Work out the finished part from the listing and answer in its coordinate system (mm). Round coordinates to 2 decimals unless told otherwise and drop trailing zeros. Loops run counter-clockwise (first coordinate to the right, second up) from the corner with the lowest first, then second, coordinate; pieces in that order, holes last. Notation, with made-up numbers: (76.5, -9.5) - (96.5, -9.5) arc R14 ccw to (96.5, 11.5) - close; hole circle Ø7 at (-30, -40). An arc over 180 degrees is marked (long way). Answer as CSV lines item,"result". Start each with the question number.
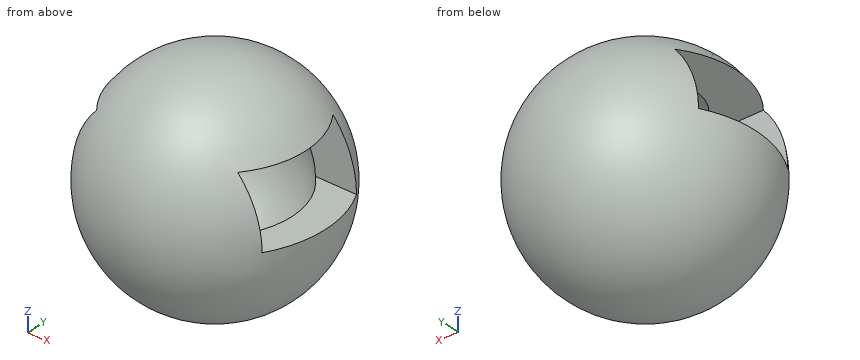
Autodesk Inventor part; units mm, degrees
ref_plane "YZ Plane" through (0, 0, 0) normal (1, 0, 0) x (0, 1, 0)
ref_plane "XZ Plane" through (0, 0, 0) normal (0, 1, 0) x (-1, 0, 0)
ref_plane "XY Plane" through (0, 0, 0) normal (0, 0, 1) x (1, 0, 0)
sketch "Эскиз1" plane through (0, 0, 0) normal (0, 0, 1) x (1, 0, 0)
  circle A0 centre (0, 0) radius 35
  line L0 (0, 35) -> (0, -35)
  dimension "d0" = 70
revolve "Вращение1" add sketch "Эскиз1" angle 360 about axis through (0, 35, 0) along (0, -1, 0)
sketch "Эскиз2" plane through (0, 0, 0) normal (1, 0, 0) x (0, 1, 0)
  circle A0 centre (-0.8026, 0) radius 25
  line L0 (24.1974, 0) -> (-25.8026, 0)
  point P0 (0, 0)
  dimension "d2" = 50
revolve "Вращение2" cut sketch "Эскиз2" angle 360 about axis through (0, 24.1974, 0) along (0, -1, 0) picked at (-3.9998, -9.7861) contours A0 L0
sketch "Эскиз3" plane through (0, 0, 0) normal (1, 0, 0) x (0, 1, 0)
  circle A0 centre (-0.8026, 0) radius 25
  line L0 (16.7899, 17.7624) -> (-18.4199, 17.7624)
  line L1 (-18.4199, 17.7624) -> (-18.4199, 0)
  line L2 (-18.4199, 0) -> (16.7899, 0)
  line L3 (16.7899, 0) -> (16.7899, 17.7624)
  line L4 (16.7899, 0) -> (-18.2101, 0)
  line L5 (-18.2101, 0) -> (-18.2101, 20)
  line L6 (-18.2101, 20) -> (16.7899, 20)
  line L7 (16.7899, 20) -> (16.7899, 0)
  point P0 (0, 0)
  dimension "d4" = 35
  dimension "d5" = 20
extrude "Выдавливание1" cut sketch "Эскиз3" along normal mid plane 100 contours L0 L5 A0 L6 | L3 L2 L5 L0 | A0 L6 L7 | A0 L5 L6
properties part number "Шар"
Item 1: Section C-C, the plane x = -3 is taken. Give the vertices of the cut face in (y, z), and give its area (3 significant figures).
Item 2: Section B-B, the plane z = 9 is taken. Give the vertices of the cut face in (x, y).
Item 3: Section A-A, the plane y = 3.5 is taken. Give the vertices of the cut face in (x, z), and give its area (3 significant figures).
Item 4: Find the intervals of material crossed by L1, parallel to Z at x = -12, y = 10.5; L2, parallel to Z at x = 21, y = -1.5; L3, parallel to Y at x = 17, z = -3, in increasing order.
Item 5: Section D-D, the plane x = -26.5 is taken. Give the vertices of the cut face in (y, z), and give its area (3 significant figures).
Item 6: Flat-ended cylindrical pins translate along their axes: pin 1 Ø16 at (x, z) = (-10.5, 14) entering from -Y; pin 2 Ø1 at (y, z) = (21.5, 1) entering from +X; pin 3 Ø3 at (y, z) = (-16, 23.5) entering from -X. Find the tip coordinate at first contact, or state that the pin passes through.
Answer:
1,outline,"circle Ø69.74 at (0, 0); hole (-18.21, 17.69) arc R24.82 ccw (long way) to (16.79, 17.51) - (16.79, 20) - (13.89, 20) arc R24.82 ccw to (-15.5, 20) - (-18.21, 20) - close"
1,area,"1,880 mm²"
2,outline,"(-29.36, 16.79) - (-15.31, 16.79) arc R23.32 cw to (15.31, 16.79) - (29.36, 16.79) arc R33.82 ccw to start; (-28.5, -18.21) arc R33.82 ccw to (28.5, -18.21) - (15.52, -18.21) arc R23.32 cw to (-15.52, -18.21) - close"
3,outline,"(-34.82, 0) arc R34.82 ccw to (34.82, 0) - (24.63, 0) arc R24.63 cw to (-24.63, 0) - close; (-28.51, 20) - (-14.37, 20) arc R24.63 cw to (14.37, 20) - (28.51, 20) arc R34.82 ccw to start"
3,area,"1,450 mm²"
4,L1,"z = -31.16 to -18.79, 20 to 31.16"
4,L2,"z = -27.96 to -13.55, 20 to 27.96"
4,L3,"y = -30.45 to -18.89, 17.28 to 30.45"
5,outline,"(-18.21, 0) - (-18.21, 13.83) arc R22.86 ccw (long way) to (16.79, 15.52) - (16.79, 0) - close; (-11.08, 20) - (11.08, 20) arc R22.86 ccw to start"
5,area,"973 mm²"
6,pin 1,"stops at y = -33.69"
6,pin 2,"stops at x = 27.98"
6,pin 3,"stops at x = -22.36"
